Job drawing, mm, ordinate dimensions from the low corner. One solid piece. Give positions to 0.01 mm unless a question says otherwise; leave off trailing zeros. Loops run counter-clockwise (first coordinate to the right, second up) from the corner with the lowest first, then second, coordinate; pieces in that order, holes last. Notation, with made-up numbers: M 78,42.25 L 94,42.25 A24 ccw 94,53.25 Z; hole C -18,-8 d3. An arc over 180 degrees is marked long. Answer in a Markdown table with one row per item.
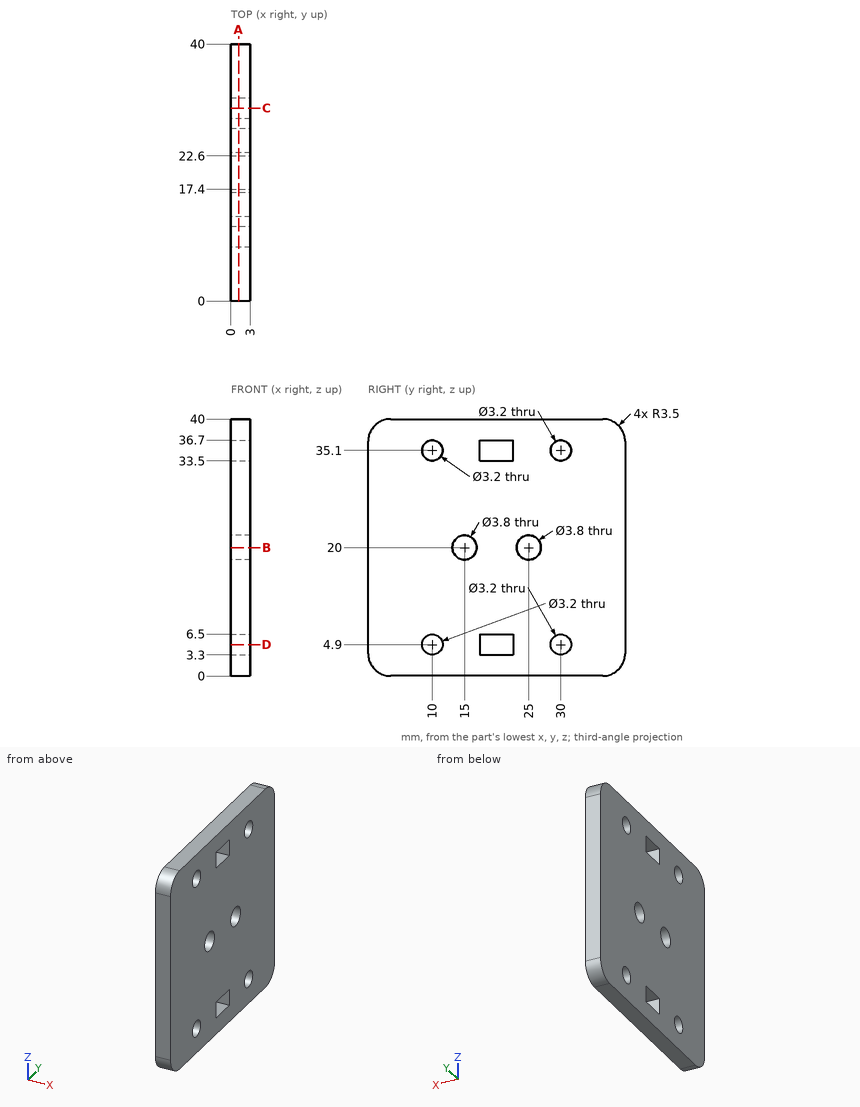
(1) Saw through at D-D (z = 4.9). Write the cut outline in (x, y), plus the area to 3 significant figures.
Recorded:
| item | result |
|---|---|
| outline | M 0,0 L 3,0 L 3,8.4 L 0,8.4 Z; M 0,11.6 L 3,11.6 L 3,17.4 L 0,17.4 Z; M 0,22.6 L 3,22.6 L 3,28.4 L 0,28.4 Z; M 0,31.6 L 3,31.6 L 3,40 L 0,40 Z |
| area | 85.2 mm^2 |
(2) Drill centre lines: line 1 along Z through (x, y) = (2.45, 10); line 2 along Y through (x, z) = (1.1, 35); line 3 along Y through (x, z) = (0.2, 6). Where is each one in solid material? Low to high.
Recorded:
| item | result |
|---|---|
| line 1 | z = 0 to 3.3, 6.5 to 33.5, 36.7 to 40 |
| line 2 | y = 0 to 8.4, 11.6 to 17.4, 22.6 to 28.4, 31.6 to 40 |
| line 3 | y = 0 to 8.84, 11.16 to 17.4, 22.6 to 28.84, 31.16 to 40 |
(3) Saw through at C-C (y = 30). Write the cut outline in (x, z).
Recorded:
| item | result |
|---|---|
| outline | M 0,0 L 3,0 L 3,3.3 L 0,3.3 Z; M 0,6.5 L 3,6.5 L 3,33.5 L 0,33.5 Z; M 0,36.7 L 3,36.7 L 3,40 L 0,40 Z |
(4) Pin check, flat tips, straight feed: pin 1 Ø8 at (y, z) = (7.5, 28.5) entering from -X; pin 2 Ø1.9 at (y, z) = (10, 35.1) entering from -X. Stop position of each tip, or through.
Recorded:
| item | result |
|---|---|
| pin 1 | stops at x = 0 |
| pin 2 | passes through |
(5) Saw through at A-A (x = 1.2). Give the number of separate pieces and of enclosed holes in the cut face, plus the area to 3 significant figures.
Recorded:
| item | result |
|---|---|
| separate pieces | 1 |
| enclosed holes | 8 |
| area | 1,500 mm^2 |
(6) Saw through at B-B (z = 20). Write the cut outline in (x, y), plus the area to 3 significant figures.
Recorded:
| item | result |
|---|---|
| outline | M 0,0 L 3,0 L 3,13.1 L 0,13.1 Z; M 0,16.9 L 3,16.9 L 3,23.1 L 0,23.1 Z; M 0,26.9 L 3,26.9 L 3,40 L 0,40 Z |
| area | 97.2 mm^2 |
